Source: three-view drawing plus pictorial views. Frame: mm from the lowest corner of the part. A direction names the side the tool comes from. Give positions to 0.01 mm unless a question says otherwise; leave off trailing zeros. Order: outer loops, then holes, each group sorted by start corner. A loop starts at its lowest first (then second) coordinate and runs counter-clockwise, first axis right, second up.
1) Draft query along Y for the marked faces 1, 2 and 3. Return one class per face: released by +Y, released by -Y, zero draft, split by the parting line, or undercut.
2) Material intervals for line 1 (Y direction, x = 24, z = 18.5); line 2 (Y direction, x = 95, z = 13.75); line 3 (X direction, y = 70.5, z = 6), sorted ascending.
3) Section C-C, the plane x = 28. Return loops of the section in (y, z), plus the area to 3 significant figures.
4) Section B-B, the plane y = 47.5. Return loops of the section in (x, z), plus the area to 3 significant figures.
5) Section A-A, the plane z = 10.5. Return loops of the section in (x, y) (3 decimals).
6) First-contact query: P1, Ø17.5, axis at x = 63, y = 67, coming from the +Z side. Flat tip, straight axial feed; report the tip coordinate or a pass-through.
7) Section D-D, the plane y = 8. Return loops of the section in (x, z).
8) Access query for the marked faces 4 and 5. Directions: +Z, -Z, +X, -X, +Y, -Y. A direction counts if a zero-diameter tool reaches every point of the face in a straight line with its end or side. Return the directions, or none.
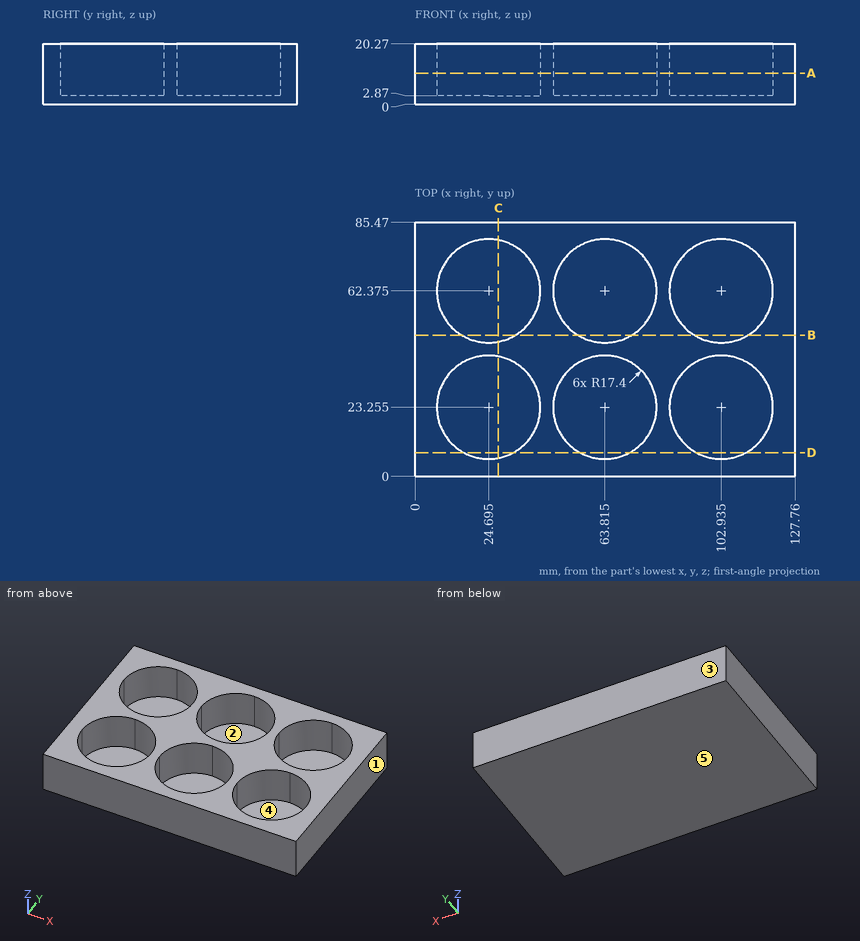
From the geometry:
1. face 1: zero draft
1. face 2: undercut
1. face 3: released by +Y
2. line 1: y = 0 to 5.87, 40.64 to 44.99, 79.76 to 85.47
2. line 2: y = 0 to 7.77, 38.74 to 46.89, 77.86 to 85.47
2. line 3: x = 0 to 9.31, 40.08 to 48.43, 79.2 to 87.55, 118.32 to 127.76
3. outline: (0, 0) - (85.47, 0) - (85.47, 20.27) - (79.46, 20.27) - (79.46, 2.87) - (45.29, 2.87) - (45.29, 20.27) - (40.34, 20.27) - (40.34, 2.87) - (6.17, 2.87) - (6.17, 20.27) - (0, 20.27) - close
3. area: 543 mm2
4. outline: (0, 0) - (127.76, 0) - (127.76, 20.27) - (111.96, 20.27) - (111.96, 2.87) - (93.91, 2.87) - (93.91, 20.27) - (72.84, 20.27) - (72.84, 2.87) - (54.79, 2.87) - (54.79, 20.27) - (33.72, 20.27) - (33.72, 2.87) - (15.67, 2.87) - (15.67, 20.27) - (0, 20.27) - close
4. area: 1,650 mm2
5. outline: (0, 0) - (127.76, 0) - (127.76, 85.47) - (0, 85.47) - close; hole circle Ø34.8 at (24.695, 23.255); hole circle Ø34.8 at (24.695, 62.375); hole circle Ø34.8 at (63.815, 23.255); hole circle Ø34.8 at (63.815, 62.375); hole circle Ø34.8 at (102.935, 23.255); hole circle Ø34.8 at (102.935, 62.375)
6. P1: stops at z = 2.87
7. outline: (0, 0) - (127.76, 0) - (127.76, 20.27) - (111.3, 20.27) - (111.3, 2.87) - (94.57, 2.87) - (94.57, 20.27) - (72.18, 20.27) - (72.18, 2.87) - (55.45, 2.87) - (55.45, 20.27) - (33.06, 20.27) - (33.06, 2.87) - (16.33, 2.87) - (16.33, 20.27) - (0, 20.27) - close
8. face 4: +Z
8. face 5: -Z, +X, -X, +Y, -Y
